Can you work these out from the model? Positions are in its coordinate system, mm. A direction names the side the tool comes from. Give positions to 0.01 mm unless a question says otherwise; leave off trailing zeros. Order: outer loops, then holes, each group sorted by start corner. A loop starts at its lowest first (then second) coordinate and runs counter-clockwise, first axis right, second up. Notation, with made-up numbers: M 33,-35.5 L 40,-35.5 A21 ccw 40,-1.5 Z; hole C 67.5,84 d7. An arc over 180 degrees is marked long. Answer as a JSON object with one key per item and string values.
Autodesk Inventor part; units mm, degrees
ref_plane "YZ Plane" through (0, 0, 0) normal (1, 0, 0) x (0, 1, 0)
ref_plane "XZ Plane" through (0, 0, 0) normal (0, 1, 0) x (-1, 0, 0)
ref_plane "XY Plane" through (0, 0, 0) normal (0, 0, 1) x (1, 0, 0)
sketch "Sketch1" plane through (0, 0, 0) normal (0, 0, 1) x (1, 0, 0)
  line L0 (-32.3125, 8) -> (32.3125, 8)
  line L1 (33.9, 6.4125) -> (33.9, -6.4125)
  line L2 (32.3125, -8) -> (-32.3125, -8)
  line L3 (-33.9, -6.4125) -> (-33.9, 6.4125)
  arc A0 (-32.3125, 8) -> (-33.9, 6.4125) centre (-32.3125, 6.4125) ccw
  arc A1 (33.9, 6.4125) -> (32.3125, 8) centre (32.3125, 6.4125) ccw
  arc A2 (32.3125, -8) -> (33.9, -6.4125) centre (32.3125, -6.4125) ccw
  arc A3 (-33.9, -6.4125) -> (-32.3125, -8) centre (-32.3125, -6.4125) ccw
  dimension "d2" = 1.5875
extrude "Extrusion1" add sketch "Sketch1" along normal blind 147
sketch "Sketch2" plane through (0, 0, 147) normal (0, 0, 1) x (1, 0, 0)
  line L0 (-28.9, 2.25) -> (-16.9, 2.25)
  line L1 (-16.9, 2.25) -> (-16.9, -2.25)
  line L2 (-16.9, -2.25) -> (-28.9, -2.25)
  line L3 (-28.9, -2.25) -> (-28.9, 2.25)
  line L4 (-28.9, 2.25) -> (-16.9, -2.25) construction
  line L5 (-16.9, 2.25) -> (-28.9, -2.25) construction
  line L6 (16.9, 2.25) -> (28.9, 2.25)
  line L7 (28.9, 2.25) -> (28.9, -2.25)
  line L8 (28.9, -2.25) -> (16.9, -2.25)
  line L9 (16.9, -2.25) -> (16.9, 2.25)
  line L10 (16.9, 2.25) -> (28.9, -2.25) construction
  line L11 (28.9, 2.25) -> (16.9, -2.25) construction
  line L12 (-33.9, 6.4125) -> (-33.9, -6.4125) construction
  line L13 (-33.9, 0) -> (33.9, 0) construction
  line L14 (33.9, -6.4125) -> (33.9, 6.4125) construction
  point P0 (0, 0)
  point P1 (-22.9, 0)
  point P2 (22.9, 0)
  dimension "d11" = 12
  dimension "d12" = 12
  dimension "d13" = 4.5
  dimension "d14" = 4.5
  dimension "d15" = 5
  dimension "d16" = 5
extrude "Extrusion2" cut sketch "Sketch2" against normal blind 10
equation "\"d16\" = d15"
properties part number "5V_LIon_speedy"
1) For faces 1 (the face through (-23, 0, 137)), 2 (the face through (-33.9, 0, 72)), which set-ups out of +Z, -Z, +X, -X, +Y, -Y let a thin tool reach every point of the face, with its end or its side?
Results found:
{"face 1": "+Z", "face 2": "+Z, -Z, -X, +Y, -Y"}
2) Thinking about a two-plate mould opening in X: for faces 3 (the face through (0, -8, 72)), 4 (the face through (-23, -2.25, 142)), 5 (the face through (33.9, 0, 72)), which applies, pulls with the +X half, pulls with the -X half, needs draft (parallel to the pull), parting line crosses it, or undercut?
Results found:
{"face 3": "needs draft", "face 4": "undercut", "face 5": "pulls with the +X half"}
3) I need wall thicknesses on L1, parallel to X at y = 1, z = 141; L2, parallel to Y at x = -25.5, z = 141; L3, parallel to Z at x = 25, y = 1.75. Which ranges of each line are inside material? Lowest first, please.
Results found:
{"L1": "x = -33.9 to -28.9, -16.9 to 16.9, 28.9 to 33.9", "L2": "y = -8 to -2.25, 2.25 to 8", "L3": "z = 0 to 137"}
4) I'm going to push flat-ended pins straight in: pin 1 Ø5 at (x, y) = (20, -0.5) entering from +Z; pin 2 Ø1.3 at (x, y) = (-22.5, 0) entering from +Z. Where does each tip first touch, or does it pass through?
Results found:
{"pin 1": "stops at z = 147", "pin 2": "stops at z = 137"}
5) I want a section at A-A on x = 22.5. Write out the boundary of the cut face in (y, z), and give its area (3 significant figures).
Results found:
{"outline": "M -8,0 L 8,0 L 8,147 L 2.25,147 L 2.25,137 L -2.25,137 L -2.25,147 L -8,147 Z", "area": "2,310 mm²"}
